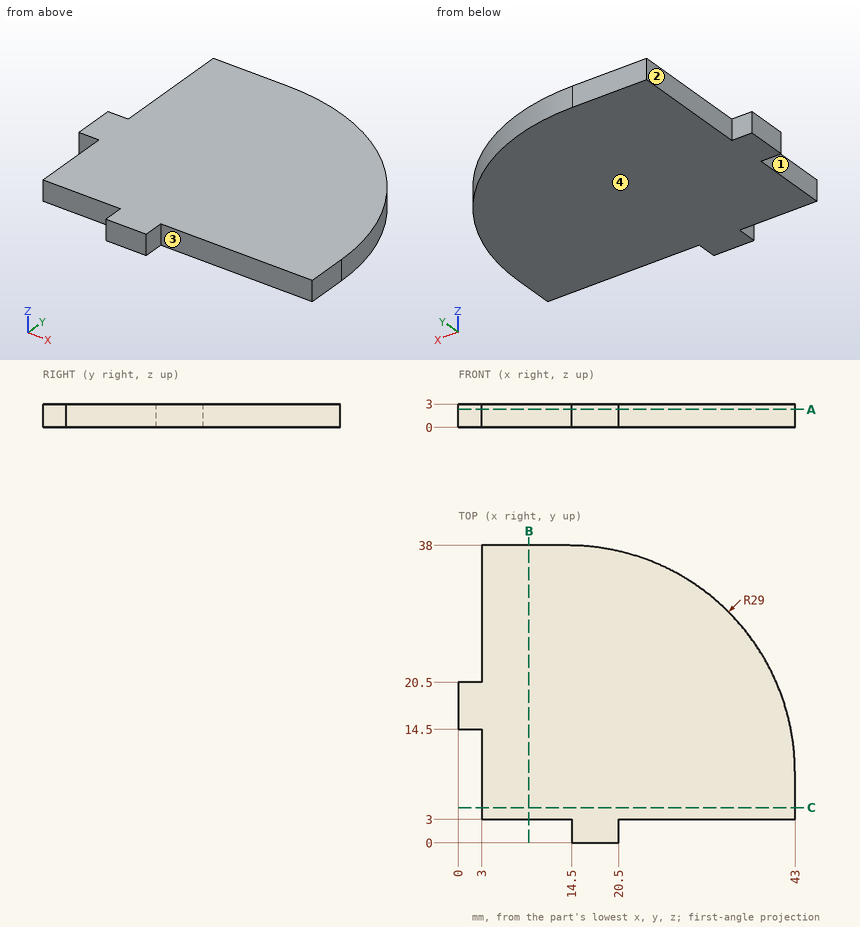
Can you work these out from the drawing? Everything is in mm from the part's minimum corner. A direction names the side the tool comes from. Round coordinates to 2 decimals unless told otherwise and drop trailing zeros. Loops run counter-clockwise (first coordinate to the right, second up) from the corner with the lowest first, then second, coordinate; pieces in that order, holes last. Notation, with made-up numbers: M -30.75,46.25 L -8.75,46.25 A31 ccw -8.75,72.25 Z; hole C -21.75,-23.75 d6. An arc over 180 degrees is marked long. Answer in a Markdown table with one row per item.
1. On a 3-axis mill with a long thin cutter (end or side, diameter ignored), from which of +Z, -Z, +X, -X, +Y, -Y can I reach the whole of each face in a straight line? I mean the marked faces 1, 2, 3 and 4. Say none if no direction works.
Established:
| item | result |
|---|---|
| face 1 | +Z, -Z, -X, -Y |
| face 2 | +Z, -Z, -X, +Y |
| face 3 | +Z, -Z, +X, -Y |
| face 4 | -Z, +X, -X, +Y, -Y |
2. If we section it at B-B, the plane x = 9: Please give me the cut outline in (y, z).
Established:
| item | result |
|---|---|
| outline | M 3,0 L 38,0 L 38,3 L 3,3 Z |
3. If we section it at C-C, the plane y = 4.5: Please give me the cut outline in (x, z), plus the area to 3 significant figures.
Established:
| item | result |
|---|---|
| outline | M 3,0 L 43,0 L 43,3 L 3,3 Z |
| area | 120 mm² |
4. Please list where these lines run through material, in increasing order: line 1 (X direction, y = 3.5, z = 1.6); line 2 (Y direction, x = 2, z = 2.9); line 3 (Y direction, x = 5, z = 1.9). Write a range as from..to.
Established:
| item | result |
|---|---|
| line 1 | 3..43 |
| line 2 | 14.5..20.5 |
| line 3 | 3..38 |
5. I'm going to push flat-ended pins straight in: pin 1 Ø1.5 at (y, z) = (29, 2) entering from -X; pin 2 Ø1.5 at (x, z) = (30.5, 1.5) entering from -Y; pin 3 Ø0.9 at (x, z) = (1.5, 1.5) entering from +Y. Where does each tip first touch, or does it pass through?
Established:
| item | result |
|---|---|
| pin 1 | x = 3 |
| pin 2 | y = 3 |
| pin 3 | y = 20.5 |
6. If we section it at A-A, the plane z = 2.3: Please give me the cut outline in (x, y), plus the area to 3 significant figures.
Established:
| item | result |
|---|---|
| outline | M 0,14.5 L 3,14.5 L 3,3 L 14.5,3 L 14.5,0 L 20.5,0 L 20.5,3 L 43,3 L 43,9 A29 ccw 14,38 L 3,38 L 3,20.5 L 0,20.5 Z |
| area | 1,260 mm² |
